Geometry check sheet. Reference: drawing and pictorial views, mm from the part's lowest x, y, z. A direction names the side the tool comes from. Give positions to 0.01 mm unless a question says otherwise; leave off trailing zeros. Loops run counter-clockwise (first coordinate to the right, second up) from the corner with the lowest first, then second, coordinate; pieces in that order, holes last. Notation, with made-up numbers: (45, -9) -> (72, -9) arc R27 ccw to (72, 11) -> close; hole circle Ø4 at (4.25, -26). An arc over 180 degrees is marked (long way). Write item = value, one per line. Start each with the question number.
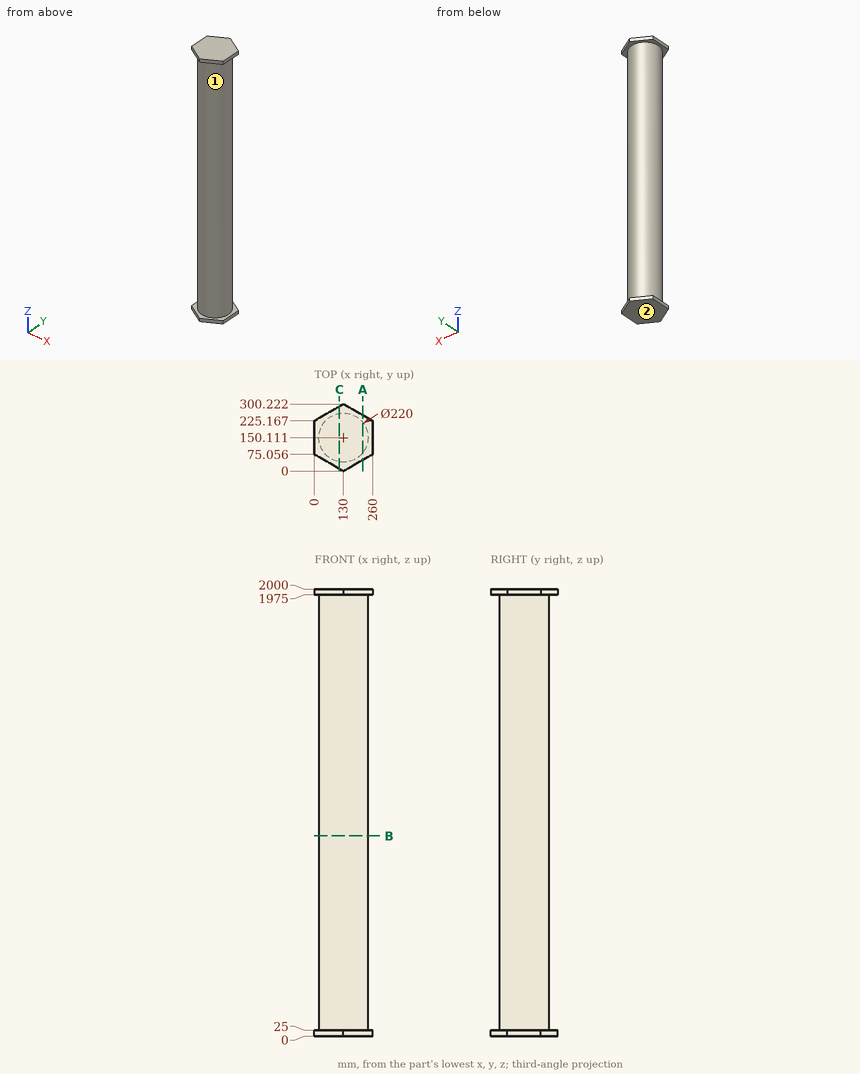
1) Tool access check on the marked faces 1 and 2. Record the directions out of +Z, -Z, +X, -X, +Y, -Y that give a thin tool (end or side, any length) a straight path to the whole face; none if there is none.
2) Section check A-A (x = 217). Enter the section's corners in (y, z), plus the area to 3 significant figures.
3) Thickness scan on line 1 (Z direction, x = 223.5, y = 59.5); line 2 (Y direction, x = 139, z = 944); line 3 (X direction, y = 152, z = 1279). Record the ranges inside material, lowest first.
4) Section check C-C (x = 111.5). Enter the section's corners in (y, z) (1 decimal), plus the area to 3 significant figures.
5) Section check B-B (z = 895.5). Enter the section's corners in (x, y).
6) Depth check by flat-ended pin: pin 1 Ø1.5 at (x, z) = (93, 895) entering from +Y; pin 2 Ø6 at (x, z) = (73.5, 1401.5) entering from -Y; pin 3 Ø1.5 at (x, z) = (103.5, 916.5) entering from +Y (1 decimal). Enter the tip coordinate at first touch or a pass-through.
Check result:
q1.face_1 = none
q1.face_2 = -Z, +X, -X, +Y, -Y
q2.outline = (50.23, 0) -> (249.99, 0) -> (249.99, 25) -> (217.42, 25) -> (217.42, 1975) -> (249.99, 1975) -> (249.99, 2000) -> (50.23, 2000) -> (50.23, 1975) -> (82.8, 1975) -> (82.8, 25) -> (50.23, 25) -> close
q2.area = 273,000 mm2
q3.line_1 = 0 to 25, 1975 to 2000
q3.line_2 = 40.48 to 259.74
q3.line_3 = 20.02 to 239.98
q4.outline = (10.7, 0) -> (289.5, 0) -> (289.5, 25) -> (258.5, 25) -> (258.5, 1975) -> (289.5, 1975) -> (289.5, 2000) -> (10.7, 2000) -> (10.7, 1975) -> (41.7, 1975) -> (41.7, 25) -> (10.7, 25) -> close
q4.area = 437,000 mm2
q5.outline = circle Ø220 at (130, 150.11)
q6.pin_1 = 253.97
q6.pin_2 = 54
q6.pin_3 = 257.1
